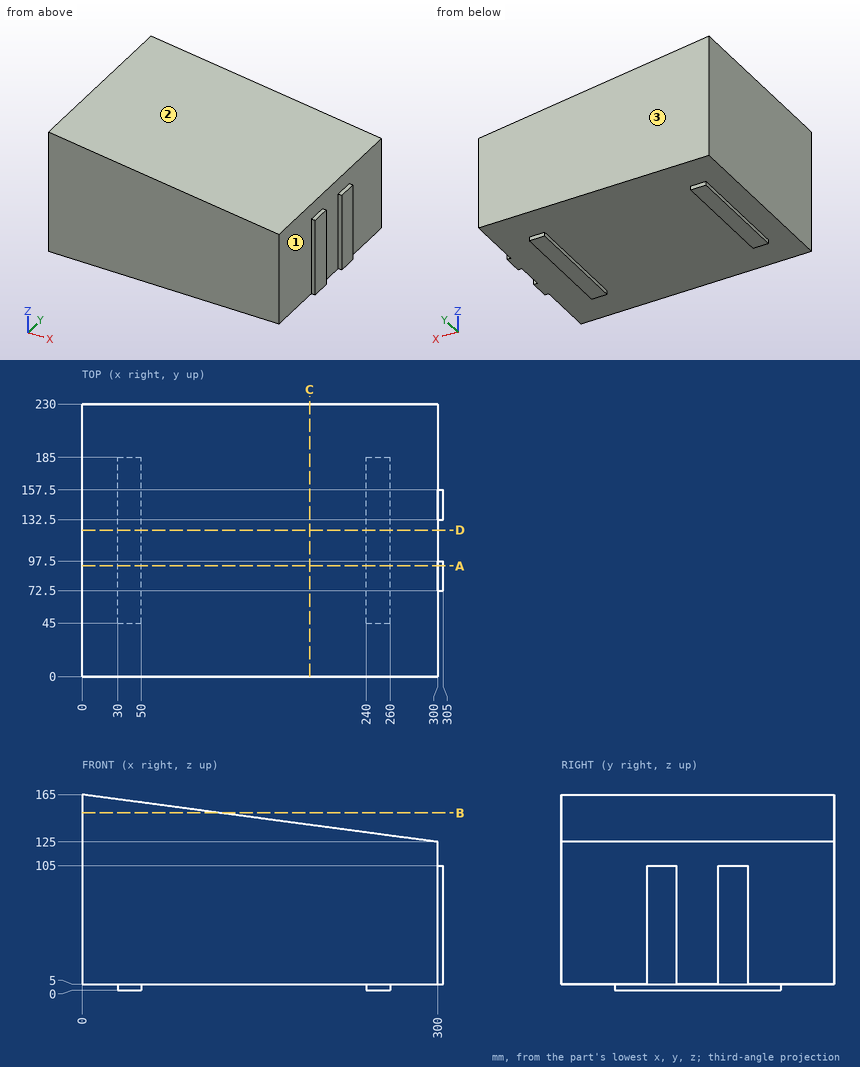
Geometry check sheet. Reference: drawing and pictorial views, mm from the part's lowest x, y, z. Coordinates: 2 decimals unless noted, no trailing zeros. Loops run counter-clockwise (first coordinate to the right, second up) from the corner with the lowest first, then second, coordinate; pieces in that order, holes last. Notation, with made-up numbers: (44.25, 74.5) -> (89.25, 74.5) arc R33 ccw to (89.25, 112.5) -> close; hole circle Ø7 at (80, 48). An arc over 180 degrees is marked (long way). Write item = value, one per line. Start each with the question number.
1. Section check B-B on z = 149.5. Record the cut outline in (x, y).
2. Section check A-A on y = 93.5. Record the cut outline in (x, z).
3. Draft check along Y on the marked faces 1, 2 and 3. Enter one of: released by +Y, released by -Y, zero draft, split by the parting line, or undercut.
4. Section check D-D on y = 123.5. Record the cut outline in (x, z).
5. Material ranges on line 1 (X direction, y = 36.5, z = 95); line 2 (Z direction, x = 150.5, y = 16); line 3 (Z direction, x = 223, y = 55), recorded low to high.
6. Section check C-C on x = 192. Record the cut outline in (y, z).
7. Depth check by flat-ended pin: P1, Ø4, axis at y = 111, z = 1.5, coming from the +X side; P2, Ø4, axis at x = 37.5, z = 2, coming from the -Y side; P3, Ø10, axis at x = 157.5, y = 150, coming from the +Z side. Enter the tip coordinate at first touch or a pass-through.
Responses:
q1.outline = (0, 0) -> (116.25, 0) -> (116.25, 230) -> (0, 230) -> close
q2.outline = (0, 5) -> (30, 5) -> (30, 0) -> (50, 0) -> (50, 5) -> (240, 5) -> (240, 0) -> (260, 0) -> (260, 5) -> (305, 5) -> (305, 105) -> (300, 105) -> (300, 125) -> (0, 165) -> close
q3.face_1 = undercut
q3.face_2 = zero draft
q3.face_3 = released by +Y
q4.outline = (0, 5) -> (30, 5) -> (30, 0) -> (50, 0) -> (50, 5) -> (240, 5) -> (240, 0) -> (260, 0) -> (260, 5) -> (300, 5) -> (300, 125) -> (0, 165) -> close
q5.line_1 = 0 to 300
q5.line_2 = 5 to 144.93
q5.line_3 = 5 to 135.27
q6.outline = (0, 5) -> (230, 5) -> (230, 139.4) -> (0, 139.4) -> close
q7.P1 = 260
q7.P2 = 45
q7.P3 = 144.67
